from build123d import *

# Parameters (mm, degrees)
BOSS_EXTRUDE1_DEPTH = 6
SKETCH2_R           = 12.59794853
CUT_EXTRUDE1_DEPTH  = 292.609327697
SKETCH3_R           = 2
CUT_EXTRUDE10_DEPTH = 292.609327697
SKETCH4_R           = 2
CUT_EXTRUDE11_DEPTH = 292.609327697
SKETCH5_R           = 2
CUT_EXTRUDE12_DEPTH = 292.609327697
SKETCH6_R           = 2
CUT_EXTRUDE13_DEPTH = 292.609327697
SKETCH8_R           = 2
CUT_EXTRUDE14_DEPTH = 292.609327697
SKETCH10_R          = 2
CUT_EXTRUDE15_DEPTH = 292.609327697
SKETCH13_W          = 33
SKETCH13_H          = 11
CUT_EXTRUDE16_DEPTH = 292.609327697


with BuildPart() as part:
    # Sketch1 → Boss-Extrude1 (new body)
    with BuildSketch(Plane(origin=(0, 0, 0), x_dir=(1, 0, 0), z_dir=(0, 1, 0))):
        with BuildLine():
            Line((0, 0), (210, 0))
            ThreePointArc((210, 0), (238.284271247, 11.715728753), (250, 40))
            Line((250, 40), (250, 110))
            ThreePointArc((250, 110), (238.284271247, 138.284271247), (210, 150))
            Line((210, 150), (0, 150))
            Line((0, 150), (0, 0))
        make_face()
    extrude(amount=BOSS_EXTRUDE1_DEPTH)

    # Sketch2 → Cut-Extrude1 (cut, through all)
    with BuildSketch(Plane.XZ):
        with Locations(Location((25, -75, 0), (0, 0, 270))):
            Circle(SKETCH2_R)
    extrude(amount=-CUT_EXTRUDE1_DEPTH, mode=Mode.SUBTRACT)

    # Sketch3 → Cut-Extrude10 (cut, through all)
    with BuildSketch(Plane(origin=(0, 6, 0), x_dir=(1, 0, 0), z_dir=(0, 1, 0))):
        with Locations(Location((6.310878228, 144.817130454, 0), (0, 0, 270))):
            Circle(SKETCH3_R)
    extrude(amount=-CUT_EXTRUDE10_DEPTH, mode=Mode.SUBTRACT)

    # Sketch4 → Cut-Extrude11 (cut, through all)
    with BuildSketch(Plane(origin=(0, 6, 0), x_dir=(1, 0, 0), z_dir=(0, 1, 0))):
        with Locations(Location((5.635720357, 4.632829204, 0), (0, 0, 270))):
            Circle(SKETCH4_R)
    extrude(amount=-CUT_EXTRUDE11_DEPTH, mode=Mode.SUBTRACT)

    # Sketch5 → Cut-Extrude12 (cut, through all)
    with BuildSketch(Plane(origin=(0, 6, 0), x_dir=(1, 0, 0), z_dir=(0, 1, 0))):
        with Locations(Location((226.364130141, 140.421237055, 0), (0, 0, 270))):
            Circle(SKETCH5_R)
    extrude(amount=-CUT_EXTRUDE12_DEPTH, mode=Mode.SUBTRACT)

    # Sketch6 → Cut-Extrude13 (cut, through all)
    with BuildSketch(Plane(origin=(0, 6, 0), x_dir=(1, 0, 0), z_dir=(0, 1, 0))):
        with Locations(Location((228.949949788, 12.164582591, 0), (0, 0, 270))):
            Circle(SKETCH6_R)
    extrude(amount=-CUT_EXTRUDE13_DEPTH, mode=Mode.SUBTRACT)

    # Sketch8 → Cut-Extrude14 (cut, through all)
    with BuildSketch(Plane(origin=(0, 6, 0), x_dir=(1, 0, 0), z_dir=(0, 1, 0))):
        with Locations(Location((242.339859996, 83, 0), (0, 0, 270))):
            Circle(SKETCH8_R)
        with Locations(Location((242.339859996, 67, 0), (0, 0, 270))):
            Circle(SKETCH8_R)
    extrude(amount=-CUT_EXTRUDE14_DEPTH, mode=Mode.SUBTRACT)

    # Sketch10 → Cut-Extrude15 (cut, through all)
    with BuildSketch(Plane(origin=(0, 6, 0), x_dir=(1, 0, 0), z_dir=(0, 1, 0))):
        with Locations(Location((50, 144.82, 0), (0, 0, 270))):
            Circle(SKETCH10_R)
        with Locations(Location((50, 4.63, 0), (0, 0, 270))):
            Circle(SKETCH10_R)
        with Locations(Location((100, 4.63, 0), (0, 0, 270))):
            Circle(SKETCH10_R)
        with Locations(Location((100, 144.82, 0), (0, 0, 270))):
            Circle(SKETCH10_R)
        with Locations(Location((50, 109.82, 0), (0, 0, 270))):
            Circle(SKETCH10_R)
        with Locations(Location((50, 39.63, 0), (0, 0, 270))):
            Circle(SKETCH10_R)
    extrude(amount=-CUT_EXTRUDE15_DEPTH, mode=Mode.SUBTRACT)

    # Sketch13 → Cut-Extrude16 (cut, through all)
    with BuildSketch(Plane(origin=(0, 6, 0), x_dir=(1, 0, 0), z_dir=(0, 1, 0))):
        with Locations((26.5, 104.5)):
            Rectangle(SKETCH13_W, SKETCH13_H)
        with Locations((26.5, 45.5)):
            Rectangle(SKETCH13_W, SKETCH13_H)
    extrude(amount=-CUT_EXTRUDE16_DEPTH, mode=Mode.SUBTRACT)


solid = part.part
Design review of the part built by this model. Coordinates are the model's own, in mm. A direction names the side the tool comes from. Give positions to 0.01 mm unless a question says otherwise; leave off trailing zeros. Loops run counter-clockwise (first coordinate to the right, second up) from the corner with the lowest first, then second, coordinate; pieces in that order, holes last. Notation, with made-up numbers: M 9.25,-2 L 51.25,-2 A12 cw 51.25,17 Z; hole C -2.75,-11 d4. An arc over 180 degrees is marked long. Write item = value, one per line.
Q1. For faces 1 (the flat face through (26, 3, -110)), 2 (the flat face through (123, 0, -76)), list the 3-axis set-ups (+Z, -Z, +X, -X, +Y, -Y) from which the entire face can be reached by the end or side of a thin tool; tool diameter is ignored.
Output values:
face_1 = +Y, -Y
face_2 = +Z, -Z, +X, -X, -Y
Q2. We need section B-B (y = 1.75). Count the separate pieces of the cut face and the enclosed holes in it, plus the area to 3 significant figures.
Output values:
separate_pieces = 1
enclosed_holes = 15
area = 35,400 mm^2
Q3. We need section A-A (z = -75). Give the boundary of the cut face in (x, y).
Output values:
outline = M 0,0 L 12.4,0 L 12.4,6 L 0,6 Z; M 37.6,0 L 250,0 L 250,6 L 37.6,6 Z
Q4. To check wall thickness, follow line 1 (X direction, y = 3.15, z = -109.82); line 2 (X direction, y = 3.9, z = -39.63); line 3 (Z direction, x = 22, y = 3.25). State the ranges of each line that lie inside material, in increasing order. Write a range as [from, to].
Output values:
line_1 = [0, 10], [43, 48], [52, 250]
line_2 = [0, 48], [52, 250]
line_3 = [-150, -110], [-99, -87.24], [-62.76, -51], [-40, 0]
Q5. Draft analysis for pull direction Z (two halves, no side actions). For faces 3 (the flat face through (104, 3, 0)), 4 (the cylindrical face through (238.594, 2.958, -137.972)), 5 (the flat face through (123, 6, -76)), 6 (the flat face through (26, 3, -51)), state which applies: +Z half, -Z half, draft (parallel to the pull), parting line (faces both ways), or undercut.
Output values:
face_3 = +Z half
face_4 = -Z half
face_5 = draft
face_6 = undercut
Q6. We need section C-C (z = -104.5). Give the boundary of the cut face in (x, y), plus the area to 3 significant figures.
Output values:
outline = M 0,0 L 10,0 L 10,6 L 0,6 Z; M 43,0 L 250,0 L 250,6 L 43,6 Z
area = 1,300 mm^2
